Design review of the part built by this model. Coordinates are the model's own, in mm. Round coordinates to 2 decimals unless told otherwise and drop trailing zeros. Order: outer loops, then holes, each group sorted by start corner. A loop starts at its lowest first (then second) coordinate and runs counter-clockwise, first axis right, second up. Notation, with made-up numbers: M 40.5,3 L 46.5,3 A34 ccw 46.5,41 Z; hole C 68,-30.75 d3. An arc over 180 degrees is marked long. Use a Markdown table: item, result. Add a question column.
(1) Take a section at A-A (x = -82.55). Write out the cut boundary in (y, z).
(2) Take a section at C-C (y = -3.75). Write out the cut boundary in (x, z).
(3) To check wall thickness, follow probe 1 along X at (y, z) = (-2, 0.5); probe 2 along Z at (x, y) = (-25, -2); probe 3 along X at (y, z) = (-2, 3). State the ranges of each line that lie inside material, in increasing order. Write a range as from..to.
(4) For pin 1 (5 mm diameter, centred on x = 26.5, z = -1, fed in from +Y), flat-tipped, find the tip position at first contact; note if it passes through.
(5) Take a section at B-B (z = 0). Write out the cut boundary in (x, y), then the cut area to 3 significant figures.
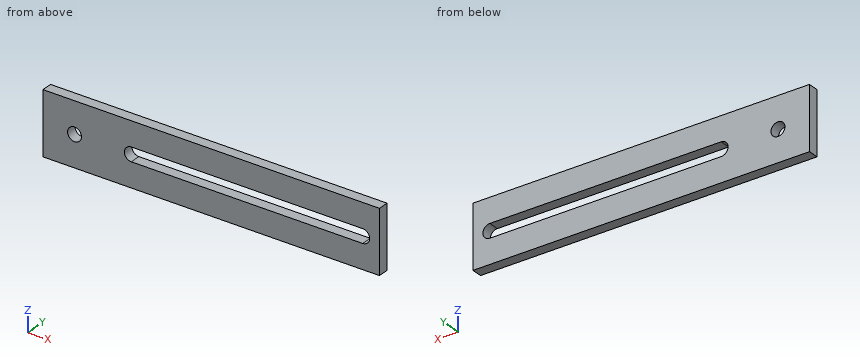
```python
from build123d import *

# Parameters (mm, degrees)
F0_W     = 203.2
F0_H     = 38.1
F1_DEPTH = 6.35
F2_R     = 4.191
F3_DEPTH = 6.35
F4_W     = 139.7
F4_H     = 8.382
F5_DEPTH = 25.4


with BuildPart() as f1:
    # F0 (on Front) → F1 (new body)
    with BuildSketch(Plane.XZ):
        Rectangle(F0_W, F0_H)
    extrude(amount=F1_DEPTH)

    # F2 (on face) → F3 (cut, through all)
    with BuildSketch(Plane.XZ.offset(6.35)):
        with Locations((-82.55, 0)):
            Circle(F2_R)
    extrude(amount=-F3_DEPTH, mode=Mode.SUBTRACT)

    # F4 (on face) → F5 (cut)
    with BuildSketch(Plane.XZ.offset(6.35)):
        with Locations((21.59, 0)):
            Rectangle(F4_W, F4_H)
        with BuildLine():
            Line((91.44, 4.191), (91.44, -4.191))
            ThreePointArc((91.44, -4.191), (95.631, 0), (91.44, 4.191))
        make_face()
        with BuildLine():
            ThreePointArc((-48.26, 4.191), (-52.451, 0), (-48.26, -4.191))
            Line((-48.26, -4.191), (-48.26, 4.191))
        make_face()
    extrude(amount=-F5_DEPTH, mode=Mode.SUBTRACT)


solid = f1.part
```
Verdict:
| question | item | result |
|---|---|---|
| 1 | outline | M -6.35,-19.05 L 0,-19.05 L 0,-4.19 L -6.35,-4.19 Z; M -6.35,4.19 L 0,4.19 L 0,19.05 L -6.35,19.05 Z |
| 2 | outline | M -101.6,-19.05 L 101.6,-19.05 L 101.6,19.05 L -101.6,19.05 Z; hole C -82.55,0 d8.38; hole M -48.26,-4.19 L 91.44,-4.19 A4.19 ccw 91.44,4.19 L -48.26,4.19 A4.19 ccw Z |
| 3 | probe 1 | x = -101.6..-86.71, -78.39..-52.42, 95.6..101.6 |
| 3 | probe 2 | z = -19.05..-4.19, 4.19..19.05 |
| 3 | probe 3 | x = -101.6..-85.48, -79.62..-51.19, 94.37..101.6 |
| 4 | pin 1 | passes through |
| 5 | outline | M -101.6,-6.35 L -86.74,-6.35 L -86.74,0 L -101.6,0 Z; M -78.36,-6.35 L -52.45,-6.35 L -52.45,0 L -78.36,0 Z; M 95.63,-6.35 L 101.6,-6.35 L 101.6,0 L 95.63,0 Z |
| 5 | area | 297 mm^2 |
